Can you work these out from the model? Positions are in its coordinate system, mm. Face numbers are marked on the shaded views. A direction names the side the tool comes from. Coordinates: 2 decimals unless noted, no trailing zeros. Order: outer loops, then holes, each group sorted by start corner. A loop starts at its lowest first (then second) coordinate and runs counter-clockwise, first axis right, second up. Notation, with made-up numbers: (78.25, 83) -> (105.25, 83) arc R17 cw to (105.25, 89) -> close; hole circle Ø11 at (61.5, 2.5). An arc over 180 degrees is marked (long way). Answer as CSV lines item,"result".
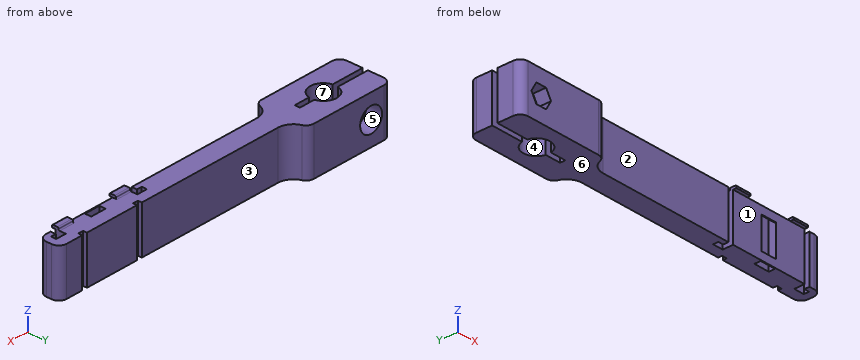
from build123d import *

# Parameters (mm, degrees)
BEAM_FOOTPRINT_DEPTH          = 18
FILLET1_R                     = 6
FILLET2_R                     = 3
FILLET3_R                     = 3
SKETCH7_R                     = 2.7
M5_BOLT_DEPTH                 = 119.105884826
SKETCH9_W                     = 6
SKETCH9_H                     = 2.8
FS_CUTOUT_DEPTH               = 6
M5_NUT_CUTOUT_DEPTH           = 5
RUBBER_BAND_NOTCH_DEPTH       = 116.784282296
RUBBER_BAND_NOTCH_DEPTH_BACK  = 116.784282296
SKETCH10_W                    = 2
SKETCH10_H                    = 1.5
WIRE_CUTOUT_DEPTH             = 117.404467388
WIRE_CUTOUT_DEPTH_BACK        = 117.404467388
SKETCH13_W                    = 6
SKETCH13_H                    = 2.4
SKETCH15_R                    = 4.6
M5_BOLT_HEAD_DEPTH            = 6
SLIDE_PLATE_CUTOUT_DEPTH      = 117.828934895
SLIDE_PLATE_CUTOUT_DEPTH_BACK = 117.828934895
SKETCH17_W                    = 6
SKETCH17_H                    = 2.5
FS_COVER_STOP_DEPTH           = 1
FILLET4_R                     = 0.4


with BuildPart() as part:
    # Sketch1 → beam footprint (new body)
    with BuildSketch(Plane.XY):
        with BuildLine():
            Line((17.5, -4), (17.5, -10))
            Line((17.5, -10), (-17.5, -10))
            Line((-17.5, -10), (-17.5, -1))
            Line((-17.5, -1), (-4.95, -1))
            ThreePointArc((-4.95, -1), (0, -5.05), (4.95, -1))
            Line((4.95, -1), (10.95, -1))
            Line((10.95, -1), (10.95, 1))
            Line((10.95, 1), (4.95, 1))
            ThreePointArc((4.95, 1), (0, 5.05), (-4.95, 1))
            Line((-4.95, 1), (-17.5, 1))
            Line((-17.5, 1), (-17.5, 10))
            Line((-17.5, 10), (17.5, 10))
            Line((17.5, 10), (17.5, 4))
            Line((17.5, 4), (115, 4))
            Line((115, 4), (115, -4))
            Line((115, -4), (17.5, -4))
        make_face()
    extrude(amount=BEAM_FOOTPRINT_DEPTH)

    # Fillet1
    fillet1_edges = [part.edges().sort_by_distance(p)[0] for p in [
        (17.5, -4, 9),
        (17.5, 4, 9),
    ]]
    fillet(fillet1_edges, radius=FILLET1_R - 0.0001)  # a hair under: the kernel refuses the full size

    # Fillet2
    fillet2_edges = [part.edges().sort_by_distance(p)[0] for p in [
        (17.5, -10, 9),
        (-17.5, -10, 9),
        (-17.5, 10, 9),
        (17.5, 10, 9),
    ]]
    fillet(fillet2_edges, radius=FILLET2_R)

    # Fillet3
    fillet3_edges = [part.edges().sort_by_distance(p)[0] for p in [
        (115, 4, 9),
        (115, -4, 9),
    ]]
    fillet(fillet3_edges, radius=FILLET3_R)

    # Sketch7 → M5 Bolt (cut, through all)
    with BuildSketch(Plane(origin=(0, 10, 0), x_dir=(1, 0, 0), z_dir=(0, 1, 0))):
        with Locations(Location((-9, -9, 0), (0, 0, 270))):
            Circle(SKETCH7_R)
    extrude(amount=-M5_BOLT_DEPTH, mode=Mode.SUBTRACT)

    # Sketch9 → FS Cutout (cut, symmetric)
    with BuildSketch(Plane.XY.offset(9)):
        with Locations((93, -2.6)):
            Rectangle(SKETCH9_W, SKETCH9_H)
    extrude(amount=FS_CUTOUT_DEPTH, both=True, mode=Mode.SUBTRACT)

    # Sketch16 → M5 Nut cutout (cut)
    with BuildSketch(Plane.XZ.offset(10)):
        Polygon((-4.9, 9), (-6.95, 12.550704156), (-11.05, 12.550704156), (-13.1, 9), (-11.05, 5.449295844), (-6.95, 5.449295844), align=None)
    extrude(amount=-M5_NUT_CUTOUT_DEPTH, mode=Mode.SUBTRACT)

    # Sketch10 → Rubber Band Notch (cut, two sides: drawn at the far end of the back side and taken through both)
    with BuildSketch(Plane.XY.offset(9).offset(-RUBBER_BAND_NOTCH_DEPTH_BACK)):
        with Locations((81.5, 3.25)):
            Rectangle(SKETCH10_W, SKETCH10_H)
        with Locations((104.5, 3.25)):
            Rectangle(SKETCH10_W, SKETCH10_H)
    extrude(amount=RUBBER_BAND_NOTCH_DEPTH + RUBBER_BAND_NOTCH_DEPTH_BACK, mode=Mode.SUBTRACT)

    # Sketch13 → Wire Cutout (cut, two sides: drawn at the far end of the back side and taken through both)
    with BuildSketch(Plane.XY.offset(3).offset(-WIRE_CUTOUT_DEPTH_BACK)):
        with Locations((93, -2.4)):
            Rectangle(SKETCH13_W, SKETCH13_H)
    extrude(amount=WIRE_CUTOUT_DEPTH + WIRE_CUTOUT_DEPTH_BACK, mode=Mode.SUBTRACT)

    # Sketch15 → M5 Bolt Head (cut)
    with BuildSketch(Plane(origin=(0, 10, 0), x_dir=(1, 0, 0), z_dir=(0, 1, 0))):
        with Locations(Location((-9, -9, 0), (0, 0, 270))):
            Circle(SKETCH15_R)
    extrude(amount=-M5_BOLT_HEAD_DEPTH, mode=Mode.SUBTRACT)

    # Sketch14 → Slide Plate Cutout (cut, two sides: drawn at the far end of the back side and taken through both)
    with BuildSketch(Plane.XY.offset(18).offset(-SLIDE_PLATE_CUTOUT_DEPTH_BACK)):
        Polygon((108, -4), (108, 0), (112, 0), (112, -2), (110, -2), (110, -4), align=None)
        Polygon((78, -4), (76, -4), (76, -2), (74, -2), (74, 0), (78, 0), align=None)
    extrude(amount=SLIDE_PLATE_CUTOUT_DEPTH + SLIDE_PLATE_CUTOUT_DEPTH_BACK, mode=Mode.SUBTRACT)

    # Sketch17 → FS cover stop (add)
    with BuildSketch(Plane.XY.offset(18)):
        with Locations((81, -4)):
            Rectangle(SKETCH17_W, SKETCH17_H)
        with Locations((105, -4)):
            Rectangle(SKETCH17_W, SKETCH17_H)
    extrude(amount=FS_COVER_STOP_DEPTH)

    # Fillet4
    fillet4_edges = [part.edges().sort_by_distance(p)[0] for p in [
        (81, -2.75, 18),
        (81, -5.25, 19),
        (81, -2.75, 19),
        (105, -2.75, 18),
        (105, -5.25, 19),
        (105, -2.75, 19),
    ]]
    fillet(fillet4_edges, radius=FILLET4_R)


solid = part.part
Q1. For P1, Ø1, axis at x = 111, z = 7.5, coming from the +Y side; P2, Ø6, axis at x = 75, y = -0.5, coming from the +Z side; P3, Ø4, axis at x = 86.5, z = 6.5, coming from the -Y side, each with a flat end and sliding along its axis, tell me the tip position at first contact or that it passes through.
Solution:
P1,"y = 4"
P2,"z = 18"
P3,"y = -4"
Q2. Which directions (+Z, -Z, +X, -X, +Y, -Y) give clear straight access to the entire face, cutting with the end or side of a thin tool? Please do the marked faces 1, 2, 3 and 4.
Solution:
face 1,"-Z, +X, -Y"
face 2,"+Z, -Z, +X, -Y"
face 3,"+Z, -Z, +X, +Y"
face 4,"+Z, -Z"
Q3. If I drill on line 1 (Y direction, x = -5, z = 16.75); line 2 (X direction, y = 2.95, z = 9); line 3 (X direction, y = -2.1, z = 9), over which ranges is the centre line in solid material (lowest first)?
Solution:
line 1,"-10 to -1, 1 to 10"
line 2,"-17.5 to -11.7, -6.3 to -4.1, 4.1 to 80.5, 82.5 to 103.5, 105.5 to 114.28"
line 3,"-17.5 to -11.7, -6.3 to -4.59, 4.59 to 76, 78 to 90, 96 to 108, 110 to 114.79"
Q4. Imagine slicing it at B-B (x = 7). List the corners of the cut face in (y, z) for me.
Solution:
outline,"(-10, 0) -> (-1, 0) -> (-1, 18) -> (-10, 18) -> close; (1, 0) -> (10, 0) -> (10, 18) -> (1, 18) -> close"
Q5. We'd pull the mould along Z, two halves only. Please class the marked faces 5, 6 and 7: pulls with the +Z half, pulls with the -Z half, needs draft (parallel to the pull), parting line crosses it, or undercut.
Solution:
face 5,"undercut"
face 6,"pulls with the -Z half"
face 7,"needs draft"
Q6. Imagine slicing it at C-C (x = 27). List the corners of the cut face in (y, z) for me.
Solution:
outline,"(-4, 0) -> (4, 0) -> (4, 18) -> (-4, 18) -> close"
Q7. Imagine slicing it at A-A (x = -9). List the corners of the cut face in (y, z) for me, and give its area (3 significant figures).
Solution:
outline,"(-10, 0) -> (-1, 0) -> (-1, 6.3) -> (-5, 6.3) -> (-5, 5.45) -> (-10, 5.45) -> close; (-10, 12.55) -> (-5, 12.55) -> (-5, 11.7) -> (-1, 11.7) -> (-1, 18) -> (-10, 18) -> close; (1, 0) -> (10, 0) -> (10, 4.4) -> (4, 4.4) -> (4, 6.3) -> (1, 6.3) -> close; (1, 11.7) -> (4, 11.7) -> (4, 13.6) -> (10, 13.6) -> (10, 18) -> (1, 18) -> close"
area,"195 mm2"
